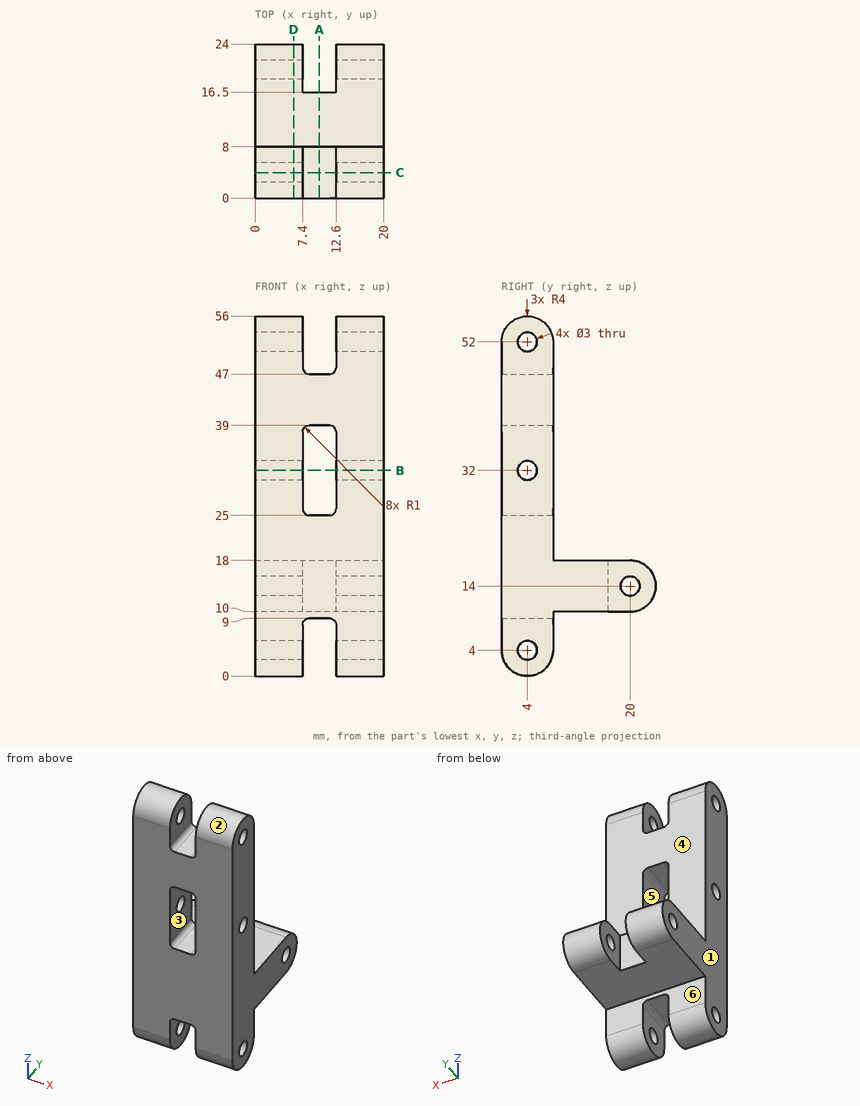
The figure shows three views and two pictorial views of one solid part (mm, origin at its lowest corner). Answer the questions. A direction names the side the tool comes from. Give positions to 0.01 mm unless a question says otherwise; leave off trailing zeros. Write each loop counter-clockwise with the first axis right and the second up, starting at its lowest first coordinate (ties: lowest second). Pieces come first, ordered by that corner, then holes. Notation, with made-up numbers: (35, -1.5) -> (88, -1.5) arc R12 cw to (88, 6.5) -> close; hole circle Ø1 at (21, -17.5). An arc over 180 degrees is marked (long way). Write each question's results on one line, items separated by ' | '.
1. Determine the mould class of the marked faces 1, 2 and 3 for opening direction X: +X half, -X half, draft (parallel to the pull), parting line (faces both ways), or undercut.
Data:
face 1: -X half | face 2: draft | face 3: undercut
2. Find section D-D on x = 6. Determine the outline of the cut face in (y, z).
Data:
outline: (0, 4) arc R4 ccw to (8, 4) -> (8, 10) -> (20, 10) arc R4 ccw to (20, 18) -> (8, 18) -> (8, 52) arc R4 ccw to (0, 52) -> close; hole circle Ø3 at (4, 4); hole circle Ø3 at (4, 32); hole circle Ø3 at (4, 52); hole circle Ø3 at (20, 14)
3. Each of these flat-tipped pins is pushed along its axis until it touches: pin 1 Ø6 at (y, z) = (11.5, 45.5) entering from +X; pin 2 Ø5.5 at (x, z) = (9.5, 15.5) entering from +Y; pin 3 Ø1.6 at (x, y) = (10, 4) entering from +Z; pin 4 Ø8 at (x, z) = (3, 35.5) entering from +Y. Where does it stop, or does it pass through?
Data:
pin 1: through | pin 2: y = 24 | pin 3: z = 47 | pin 4: y = 8
4. Find section C-C on y = 4. Give the number of separate pieces and of enclosed holes in the cut face, and give its area (3 significant figures).
Data:
separate pieces: 6 | enclosed holes: 0 | area: 822 mm^2
5. Straight lines are drawn through the part: L1, parallel to Z at x = 3.75, y = 4; L2, parallel to X at y = 5, z = 29; L3, parallel to Z at x = 11.5, y = 6.75. For each, find the intervals that lie inside material, in ascending order.
Data:
L1: 0 to 2.5, 5.5 to 30.5, 33.5 to 50.5, 53.5 to 56 | L2: 0 to 7.4, 12.6 to 20 | L3: 9 to 25, 39 to 47
6. Find section A-A on x = 10. Determine the outline of the cut face in (y, z), and give its area (3 significant figures).
Data:
outline: (0, 9) -> (8, 9) -> (8, 10) -> (16.5, 10) -> (16.5, 18) -> (8, 18) -> (8, 25) -> (0, 25) -> close; (0, 39) -> (8, 39) -> (8, 47) -> (0, 47) -> close | area: 260 mm^2
7. Find section B-B on z = 32. Determine the outline of the cut face in (x, y).
Data:
outline: (0, 0) -> (7.4, 0) -> (7.4, 2.5) -> (0, 2.5) -> close; (0, 5.5) -> (7.4, 5.5) -> (7.4, 8) -> (0, 8) -> close; (12.6, 0) -> (20, 0) -> (20, 2.5) -> (12.6, 2.5) -> close; (12.6, 5.5) -> (20, 5.5) -> (20, 8) -> (12.6, 8) -> close
8. A tool of negligible diameter and unlimited length cuts with its end or side. For the marked faces 4, 5 and 6, from which of +Z, -Z, +X, -X, +Y, -Y can it reach the whole face along a straight path? Write none if from no direction.
Data:
face 4: +Z, +X, -X, +Y | face 5: +Y, -Y | face 6: -Z, +X, -X, +Y
